```python
from build123d import *

# Parameters (mm, degrees)
SKETCH_1_W                  = 230
SKETCH_1_H                  = 84.29
EXTRUDE_1_DEPTH             = 3
EXTRUDE_2_DEPTH             = 3
EXTRUDE_2_DEPTH_BACK        = 233
SKETCH_3_W                  = 3
SKETCH_3_H                  = 35
SKETCH_2_R                  = 2
CUT_EXTRUDE_1_DEPTH         = 3
SKETCH_5_R                  = 1.5
CUT_EXTRUDE_2_DEPTH         = 3
SKETCH_6_W                  = 3
SKETCH_6_H                  = 25
CUT_EXTRUDE_3_DEPTH         = 3
CUT_EXTRUDE_4_DEPTH         = 3
SKETCH_8_W                  = 30
SKETCH_8_H                  = 3
EXTRUDE_3_DEPTH             = 5
FILLET_1_R                  = 5
FILLET_2_R                  = 5
SKETCH_9_R                  = 1.5
CUT_EXTRUDE_5_DEPTH         = 10
SKETCH_10_R                 = 8
CUT_EXTRUDE_6_DEPTH         = 10
SKETCH_11_W                 = 10
SKETCH_11_H                 = 4.5
CUT_EXTRUDE_7_DEPTH         = 10
FILLET_3_R                  = 1.5
SKETCH_12_R                 = 1.5
CUT_EXTRUDE_8_DEPTH         = 10
PATTERN_LINEAR_1_COUNT      = 7
PATTERN_LINEAR_1_PITCH      = 20
PATTERN_LINEAR_1_COUNT_DIR2 = 4
PATTERN_LINEAR_1_PITCH_DIR2 = 8


with BuildPart() as part:
    # Эскиз1 → Бобышка-Вытянуть1 (new body)
    with BuildSketch(Plane.XY):
        with Locations((115, 42.145)):
            Rectangle(SKETCH_1_W, SKETCH_1_H)
    extrude(amount=EXTRUDE_1_DEPTH)

    # Эскиз3 → Бобышка-Вытянуть2 (add, two sides: drawn at the far end of the back side and taken through both)
    with BuildSketch(Plane(origin=(230, 0, 0), x_dir=(0, 0, -1), z_dir=(1, 0, 0)).offset(-EXTRUDE_2_DEPTH_BACK)):
        with Locations((-1.5, 42.145)):
            Rectangle(SKETCH_3_W, SKETCH_3_H)
    extrude(amount=EXTRUDE_2_DEPTH + EXTRUDE_2_DEPTH_BACK)

    # Эскиз2 → Вырез-Вытянуть1 (cut)
    with BuildSketch(Plane.XY.offset(3)):
        with Locations((65, 40.4)):
            Circle(SKETCH_2_R)
        with Locations((165, 40.4)):
            Circle(SKETCH_2_R)
    extrude(amount=-CUT_EXTRUDE_1_DEPTH, mode=Mode.SUBTRACT)

    # Эскиз5 → Вырез-Вытянуть2 (cut)
    with BuildSketch(Plane.XY.offset(3)):
        with Locations((33.5, 70)):
            Circle(SKETCH_5_R)
        with Locations((33.5, 20)):
            Circle(SKETCH_5_R)
        with Locations((196.5, 20)):
            Circle(SKETCH_5_R)
        with Locations((196.5, 70)):
            Circle(SKETCH_5_R)
    extrude(amount=-CUT_EXTRUDE_2_DEPTH, mode=Mode.SUBTRACT)

    # Эскиз6 → Вырез-Вытянуть3 (cut)
    with BuildSketch(Plane.XY.offset(3)):
        with Locations((33.5, 45)):
            Rectangle(SKETCH_6_W, SKETCH_6_H)
        with Locations((196.5, 45)):
            Rectangle(SKETCH_6_W, SKETCH_6_H)
    extrude(amount=-CUT_EXTRUDE_3_DEPTH, mode=Mode.SUBTRACT)

    # Эскиз7 → Вырез-Вытянуть4 (cut)
    with BuildSketch(Plane.XY.offset(3)):
        Polygon((0, 73.4675), (6, 73.4675), (6, 74.7175), (8.5, 74.7175), (8.5, 73.4675), (14.5, 73.4675), (14.5, 70.4675), (8.5, 70.4675), (8.5, 69.2175), (6, 69.2175), (6, 70.4675), (0, 70.4675), align=None)
        Polygon((0, 13.8225), (0, 10.8225), (6, 10.8225), (6, 9.5725), (8.5, 9.5725), (8.5, 10.8225), (14.5, 10.8225), (14.5, 13.8225), (8.5, 13.8225), (8.5, 15.0725), (6, 15.0725), (6, 13.8225), align=None)
        Polygon((230, 10.8225), (224, 10.8225), (224, 9.5725), (221.5, 9.5725), (221.5, 10.8225), (215.5, 10.8225), (215.5, 13.8225), (221.5, 13.8225), (221.5, 15.0725), (224, 15.0725), (224, 13.8225), (230, 13.8225), align=None)
        Polygon((230, 70.4675), (230, 73.4675), (224, 73.4675), (224, 74.7175), (221.5, 74.7175), (221.5, 73.4675), (215.5, 73.4675), (215.5, 70.4675), (221.5, 70.4675), (221.5, 69.2175), (224, 69.2175), (224, 70.4675), align=None)
    extrude(amount=-CUT_EXTRUDE_4_DEPTH, mode=Mode.SUBTRACT)

    # Эскиз8 → Бобышка-Вытянуть3 (add)
    with BuildSketch(Plane(origin=(0, 84.29, 0), x_dir=(1, 0, 0), z_dir=(0, 1, 0))):
        with Locations((15, -1.5)):
            Rectangle(SKETCH_8_W, SKETCH_8_H)
    extrude(amount=EXTRUDE_3_DEPTH)

    # Скругление1
    fillet_1_edges = [part.edges().sort_by_distance(p)[0] for p in [
        (30, 89.29, 1.5),
    ]]
    fillet(fillet_1_edges, radius=FILLET_1_R - 0.0001)  # a hair under: the kernel refuses the full size

    # Скругление2
    fillet_2_edges = [part.edges().sort_by_distance(p)[0] for p in [
        (30, 84.29, 1.5),
    ]]
    fillet(fillet_2_edges, radius=FILLET_2_R)

    # Эскиз9 → Вырез-Вытянуть5 (cut)
    with BuildSketch(Plane(origin=(0, 0, 0), x_dir=(-1, 0, 0), z_dir=(0, 0, -1))):
        with Locations((-180, 65.4)):
            Circle(SKETCH_9_R)
        with Locations((-50, 65.4)):
            Circle(SKETCH_9_R)
        with Locations((-115, 55.4)):
            Circle(SKETCH_9_R)
    extrude(amount=-CUT_EXTRUDE_5_DEPTH, mode=Mode.SUBTRACT)

    # Эскиз10 → Вырез-Вытянуть6 (cut)
    with BuildSketch(Plane(origin=(0, 0, 0), x_dir=(-1, 0, 0), z_dir=(0, 0, -1))):
        with Locations((-185, 50.5)):
            Circle(SKETCH_10_R)
        with Locations((-129, 50.5)):
            Circle(SKETCH_10_R)
        with Locations((-101, 50.5)):
            Circle(SKETCH_10_R)
        with Locations((-45, 50.5)):
            Circle(SKETCH_10_R)
    extrude(amount=-CUT_EXTRUDE_6_DEPTH, mode=Mode.SUBTRACT)

    # Эскиз11 → Вырез-Вытянуть7 (cut)
    with BuildSketch(Plane(origin=(0, 0, 0), x_dir=(-1, 0, 0), z_dir=(0, 0, -1))):
        with Locations((-155, 63.25)):
            Rectangle(SKETCH_11_W, SKETCH_11_H)
        with Locations((-75, 63.25)):
            Rectangle(SKETCH_11_W, SKETCH_11_H)
        with Locations((-75, 70.75)):
            Rectangle(SKETCH_11_W, SKETCH_11_H)
        with Locations((-155, 70.75)):
            Rectangle(SKETCH_11_W, SKETCH_11_H)
    extrude(amount=-CUT_EXTRUDE_7_DEPTH, mode=Mode.SUBTRACT)

    # Скругление3
    fillet_3_edges = [part.edges().sort_by_distance(p)[0] for p in [
        (160, 61, 1.5),
        (160, 65.5, 1.5),
        (150, 65.5, 1.5),
        (150, 61, 1.5),
        (80, 61, 1.5),
        (80, 65.5, 1.5),
        (70, 65.5, 1.5),
        (70, 61, 1.5),
        (70, 73, 1.5),
        (70, 68.5, 1.5),
        (80, 68.5, 1.5),
        (80, 73, 1.5),
        (150, 73, 1.5),
        (150, 68.5, 1.5),
        (160, 68.5, 1.5),
        (160, 73, 1.5),
    ]]
    fillet(fillet_3_edges, radius=FILLET_3_R)

    # Эскиз12 → Вырез-Вытянуть8 (cut)
    with BuildSketch(Plane.XY.offset(3)):
        with Locations((55, 8)):
            Circle(SKETCH_12_R)
    cut_extrude_8 = extrude(amount=-CUT_EXTRUDE_8_DEPTH, mode=Mode.SUBTRACT)

    # Линейный массив1: Cut-Extrude 8 7 × 4
    with Locations(*[(i * PATTERN_LINEAR_1_PITCH, j * PATTERN_LINEAR_1_PITCH_DIR2, 0) for i in range(PATTERN_LINEAR_1_COUNT) for j in range(PATTERN_LINEAR_1_COUNT_DIR2) if (i, j) != (0, 0)]):
        add(cut_extrude_8, mode=Mode.SUBTRACT)


solid = part.part
```
Read the model definition and answer for the solid it produces. Units are mm, in the model's axes. Give positions to 0.01 mm unless a question says otherwise; leave off trailing zeros. Order: outer loops, then holes, each group sorted by start corner. A loop starts at its lowest first (then second) coordinate and runs counter-clockwise, first axis right, second up.
(1) Given pin 1 (0.9 mm diameter, centred on y = 63, z = 2, fed in from -X); pin 2 (1.5 mm diameter, centred on x = 218.5, z = 1.5, fed in from +Y); pin 3 (1.6 mm diameter, centred on y = 71, z = 1.5, fed in from +X), each flat-ended and moving along its own axis, determine where each tip first touches the part or whether it passes through.
(2) For a pull along X with two mould halves and no side action, classify faces 1 (the cylindrical face through (50.9, 55.9, 1.5)), 2 (the flat face through (113, 44, 3)) as released by +X, released by -X, zero draft, split by the parting line, or undercut.
(3) Straight lines are drawn through the part: L1, parallel to X at y = 40, z = 1.5; L2, parallel to Y at x = 157, z = 0.8; L3, parallel to Y at x = 55, z = 1.2. For each, find the intervals that lie inside material, in ascending order.
(4) Find section A-A (x = 89). Give the vertices of the cut face in (y, z), plus the area to 3 significant figures.
(5) Find section B-B (z = 2.15). Give the number of separate pieces and of enclosed holes in the cut face, plus the area to 3 significant figures.
Result sheet:
1. pin 1: stops at x = 0
1. pin 2: stops at y = 84.29
1. pin 3: stops at x = 230
2. face 1: undercut
2. face 2: zero draft
3. L1: x = -3 to 32, 35 to 63.04, 66.96 to 163.04, 166.96 to 195, 198 to 233
3. L2: y = 0 to 61, 65.5 to 68.5, 73 to 84.29
3. L3: y = 0 to 6.5, 9.5 to 14.5, 17.5 to 22.5, 25.5 to 30.5, 33.5 to 84.29
4. outline: (0, 0) - (84.29, 0) - (84.29, 3) - (0, 3) - close
4. area: 253 mm2
5. separate pieces: 1
5. enclosed holes: 47
5. area: 18,100 mm2
